Geometry: final body of the model. Coordinates: model frame, mm. Face numbers are marked on the shaded views. A direction names the side the tool comes from. Coordinates: 2 decimals unless noted, no trailing zeros. Order: outer loops, then holes, each group sorted by start corner. A loop starts at its lowest first (then second) coordinate and runs counter-clockwise, first axis right, second up. Notation, with made-up numbers: (81.5, 86.5) - (129.5, 86.5) arc R16 ccw to (129.5, 97.5) - close; hole circle Ø2 at (20, -10.5). An arc over 180 degrees is marked (long way). Use a Markdown table: item, result. Add a question column.
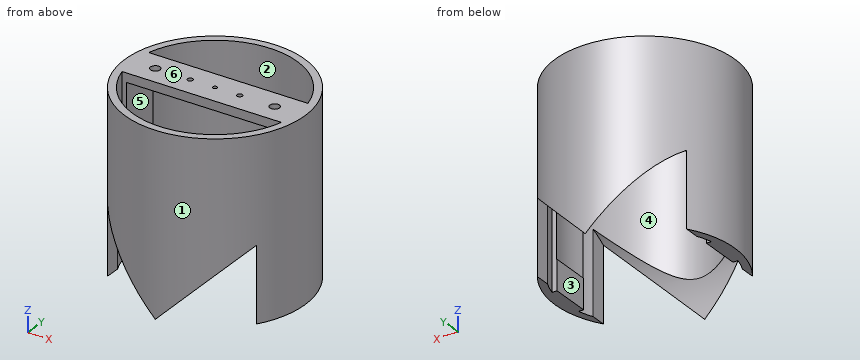
Autodesk Inventor part; units mm, degrees
ref_plane "YZ Plane" through (0, 0, 0) normal (1, 0, 0) x (0, 1, 0)
ref_plane "XZ Plane" through (0, 0, 0) normal (0, 1, 0) x (-1, 0, 0)
ref_plane "XY Plane" through (0, 0, 0) normal (0, 0, 1) x (1, 0, 0)
sketch "スケッチ1" plane through (0, 0, 0) normal (0, 0, 1) x (1, 0, 0)
  circle A0 centre (0, 0) radius 30
  dimension "d0" = 60
extrude "押し出し1" add sketch "スケッチ1" along normal blind 60
sketch "スケッチ2" plane through (0, 0, 60) normal (0, 0, 1) x (1, 0, 0)
  circle A0 centre (0, 0) radius 26
  dimension "d3" = 52
extrude "押し出し2" cut sketch "スケッチ2" against normal blind 50
sketch "スケッチ3" plane through (0, 0, 0) normal (0, 0, 1) x (1, 0, 0)
  point P0 (0, 0)
sketch "スケッチ4" plane through (0, 0, 0) normal (1, 0, 0) x (0, 1, 0)
  line L0 (30, 0) -> (-30, 0)
  line L1 (-30, 0) -> (-30, 60)
  arc A0 (30, 0) -> (-30, 0) centre (0, 0) ccw
  dimension "d6" = 30
extrude "押し出し3" cut sketch "スケッチ4" along normal mid plane 50
sketch "スケッチ5" plane through (0, 0, 60) normal (0, 0, 1) x (1, 0, 0)
  circle A0 centre (0, 0) radius 27.5
extrude "押し出し4" add sketch "スケッチ5" against normal blind 3
sketch "スケッチ19" plane through (0, 0, 60) normal (0, 0, 1) x (1, 0, 0)
  circle A0 centre (0, 0) radius 27.5
  line L0 (27.5, -6.6575) -> (-27.5, -6.6575)
  line L1 (-27.5, -6.6575) -> (-27.5, 6.6575)
  line L2 (-27.5, 6.6575) -> (27.5, 6.6575)
  line L3 (27.5, 6.6575) -> (27.5, -6.6575)
  line L4 (27.5, -6.6575) -> (-27.5, 6.6575) construction
  line L5 (-27.5, -6.6575) -> (27.5, 6.6575) construction
  point P0 (26.682, -6.6575)
  point P1 (-26.682, -6.6575)
  point P2 (-26.682, 6.6575)
  point P3 (26.682, 6.6575)
extrude "押し出し11" cut sketch "スケッチ19" against normal blind 60 contours L2 A0 | A0 L0
sketch "スケッチ22" plane through (0, 0, 60) normal (0, 0, 1) x (1, 0, 0)
  point P0 (0, 0)
sketch "スケッチ23" plane through (0, 0, 60) normal (0, 0, 1) x (1, 0, 0)
  point P0 (0, 0)
  point P1 (-20, 0)
  point P2 (20, 0)
  dimension "d67" = 20
  dimension "d68" = 20
hole "穴4" at (-20, 0, 60) at (20, 0, 60) direction (0, 0, -1) diameter 3.2 depth 8.8 tip angle 118
sketch "スケッチ25" plane through (0, 0, 60) normal (0, 0, 1) x (1, 0, 0)
  point P0 (0, 0)
  point P1 (0, 0)
hole "穴5" at (0, 0, 60) direction (0, 0, -1) diameter 1.5 depth 8.8 tip angle 118
sketch "スケッチ27" plane through (0, 0, 57) normal (0, 0, -1) x (-1, 0, 0)
  point P0 (0, 0)
  point P1 (8.3, 0)
  point P2 (-8.3, 0)
  dimension "d95" = 8.3
  dimension "d96" = 8.3
hole "穴7" at (-8.3, 0, 57) at (8.3, 0, 57) direction (0, 0, 1) diameter 1.8 depth 8.8 tip angle 118 counterbore diameter 4 counterbore depth 2
properties part number "20220527_仮筒"
1) Section query D-D (x = -2). Return the cut outline in (y, z).
2) Section query C-C (z = 8). Return the cut outline in (x, y), and give its area (3 significant figures).
3) Draft query along Y for the marked faces 1, 2 and 3. Return one class per face: released by +Y, released by -Y, zero draft, split by the parting line, or undercut.
4) Line query: line 1 (Y direction, x = 1, z = 36); line 2 (Y direction, x = -7, z = 57.5); line 3 (Y direction, x = -25, z = 32). Output: solid intervals per line, ascending. Write a range as from..to.
5) First-contact query: pin 1 (2.5 mm diameter, centred on x = -8.3, y = 0, fed in from -Z); pin 2 (1.5 mm diameter, centred on x = -10, z = 10.5, fed in from +Y); pin 3 (1.5 mm diameter, centred on y = -13, z = 15.5, fed in from -X) (3 decimals); pin 4 (5 mm diameter, centred on y = -1, z = 3, fed in from -X). Flat tips, straight axial feed; report the tip coordinate or a pass-through.
6) Access query for the marked faces 4, 5 and 6. Directions: +Z, -Z, +X, -X, +Y, -Y. A direction counts if a zero-diameter tool reaches every point of the face in a straight line with its end or side. Return the directions, or none.
7) Section query B-B (y = -9.5). Return the cut outline in (x, z), and give its area (3 significant figures).
8) Section query A-A (z = 37.5). Return the cut outline in (x, y), and give its area (3 significant figures).
From the geometry:
| question | item | result |
|---|---|---|
| 1 | outline | (-29.93, 2) arc R30 cw to (-27.43, 12.16) - (-27.43, 60) - (-29.93, 60) - close; (-6.66, 57) - (6.66, 57) - (6.66, 60) - (-6.66, 60) - close; (27.43, 12.16) arc R30 cw to (29.93, 2) - (29.93, 60) - (27.43, 60) - close |
| 2 | outline | (-26.68, -6.66) - (-25, -6.66) - (-25, 6.66) - (-26.68, 6.66) arc R27.5 cw to (-25, 11.46) - (-25, 16.58) arc R30 ccw to (-25, -16.58) - (-25, -11.46) arc R27.5 cw to start; (-8, -28.91) arc R30 ccw to (8, -28.91) - close; (-8, 28.91) - (8, 28.91) arc R30 ccw to start; (25, -16.58) arc R30 ccw to (25, 16.58) - (25, 11.46) arc R27.5 cw to (26.68, 6.66) - (25, 6.66) - (25, -6.66) - (26.68, -6.66) arc R27.5 cw to (25, -11.46) - close |
| 2 | area | 231 mm^2 |
| 3 | face 1 | split by the parting line |
| 3 | face 2 | undercut |
| 3 | face 3 | zero draft |
| 4 | line 1 | y = -29.98..-27.48, 27.48..29.98 |
| 4 | line 2 | y = -29.17..-26.59, -6.66..-1.52, 1.52..6.66, 26.59..29.17 |
| 4 | line 3 | y = -16.58..-11.46, 11.46..16.58 |
| 5 | pin 1 | stops at z = 59 |
| 5 | pin 2 | stops at y = 28.54 |
| 5 | pin 3 | stops at x = -27.385 |
| 5 | pin 4 | stops at x = -30 |
| 6 | face 4 | +Z, -Z |
| 6 | face 5 | none |
| 6 | face 6 | +Z, +X, -X, +Y, -Y |
| 7 | outline | (-28.46, 0) - (-25.81, 0) - (-25.81, 60) - (-28.46, 60) - close; (25.81, 0) - (28.46, 0) - (28.46, 60) - (25.81, 60) - close |
| 7 | area | 318 mm^2 |
| 8 | outline | circle Ø60 at (0, 0); hole (-26.68, -6.66) arc R27.5 ccw to (26.68, -6.66) - (25.13, -6.66) arc R26 ccw to (25.13, 6.66) - (26.68, 6.66) arc R27.5 ccw to (-26.68, 6.66) - (-25.13, 6.66) arc R26 ccw to (-25.13, -6.66) - close |
| 8 | area | 492 mm^2 |
